For this review, use the dimensioned drawing (mm, ordinates from the lowest corner) and the shaded views. A direction names the side the tool comes from. Coordinates: 2 decimals unless noted, no trailing zeros. Write each loop counter-clockwise with the first axis right and the second up, starting at its lowest first coordinate (ties: lowest second). Pieces come first, ordered by that corner, then holes. Notation, with made-up numbers: (-32, -33) - (14, -33) arc R20 cw to (14, -7) - close; hole circle Ø10 at (27.25, 39.25). An arc over 180 degrees is marked (long way). Answer as a JSON object with one key per item and string values.
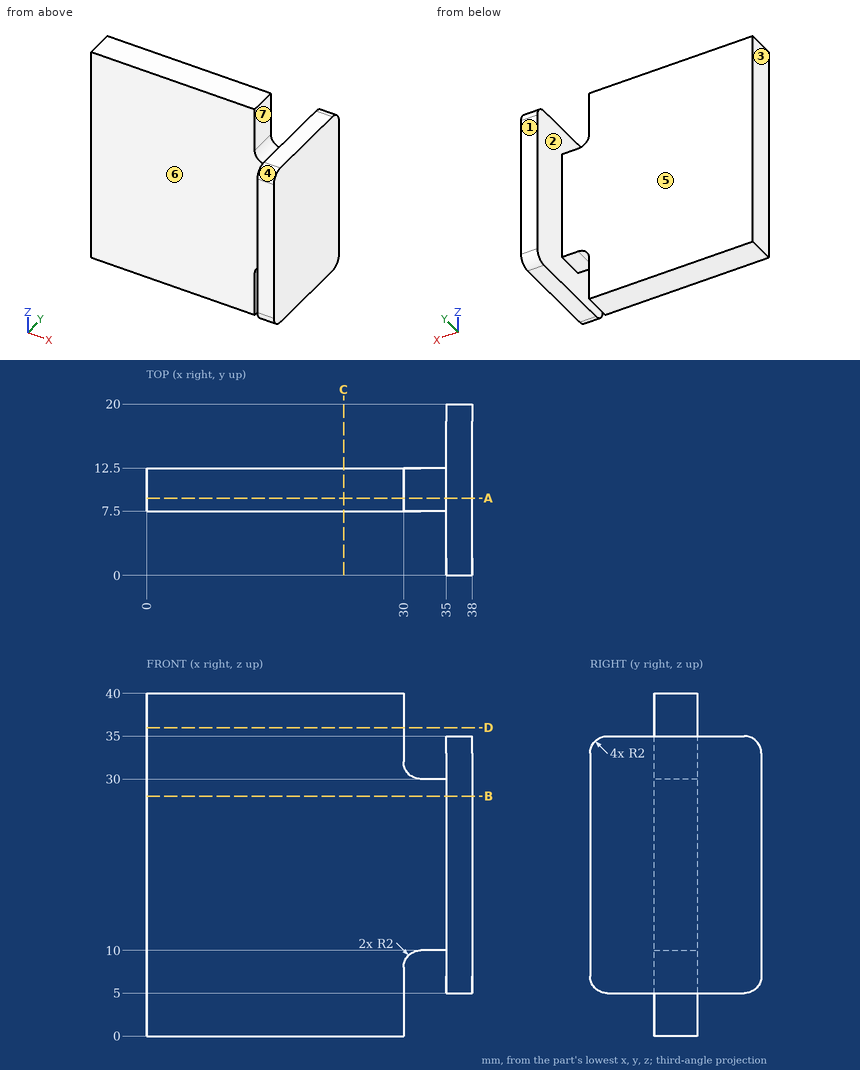
(1) Take a section at A-A, the plane y = 9. Write out the cut boundary in (x, z).
Solved:
{"outline": "(0, 0) - (30, 0) - (30, 8) arc R2 cw to (32, 10) - (35, 10) - (35, 5) - (38, 5) - (38, 35) - (35, 35) - (35, 30) - (32, 30) arc R2 cw to (30, 32) - (30, 40) - (0, 40) - close"}
(2) Take a section at D-D, the plane z = 36. Write out the cut boundary in (x, y).
Solved:
{"outline": "(0, 7.5) - (30, 7.5) - (30, 12.5) - (0, 12.5) - close"}
(3) Take a section at B-B, the plane z = 28. Write out the cut boundary in (x, y), and give its area (3 significant figures).
Solved:
{"outline": "(0, 7.5) - (35, 7.5) - (35, 0) - (38, 0) - (38, 20) - (35, 20) - (35, 12.5) - (0, 12.5) - close", "area": "235 mm^2"}
(4) To check wall thickness, follow line 1 (Y direction, x = 15.5, z = 21.5); line 2 (X direction, y = 17.25, z = 27); line 3 (Z direction, x = 36.5, y = 9). State the ranges of each line that lie inside material, in increasing order. Write a range as from..to.
Solved:
{"line 1": "y = 7.5..12.5", "line 2": "x = 35..38", "line 3": "z = 5..35"}
(5) Tool access review of the marked faces 4, 5, 6 and 7: name each direction out of +Z, -Z, +X, -X, +Y, -Y from which nothing blocks a thin tool from reaching the whole face with its end or side.
Solved:
{"face 4": "+Z, +X, -X, -Y", "face 5": "+Z, -Z, -X, +Y", "face 6": "+Z, -Z, -X, -Y", "face 7": "+Z, +Y, -Y"}
(6) The part is to be moulded in two halves that separate along X. For the marked faces 1, 2 and 3, say which applies: pulls with the +X half, pulls with the -X half, needs draft (parallel to the pull), parting line crosses it, or undercut.
Solved:
{"face 1": "needs draft", "face 2": "undercut", "face 3": "pulls with the -X half"}
(7) For pin 1 (6 mm diameter, centred on x = 5, z = 31, fed in from +Y); pin 2 (5 mm diameter, centred on x = 7, z = 36, fed in from -Y); pin 3 (0.9 mm diameter, centred on x = 34, y = 10.5, fed in from +Z), all flat-tipped, find the tip position at first contact; note any pin that passes through.
Solved:
{"pin 1": "stops at y = 12.5", "pin 2": "stops at y = 7.5", "pin 3": "stops at z = 30"}
(8) Take a section at C-C, the plane x = 23. Write out the cut boundary in (y, z), and give its area (3 significant figures).
Solved:
{"outline": "(7.5, 0) - (12.5, 0) - (12.5, 40) - (7.5, 40) - close", "area": "200 mm^2"}
